Part model, mm, in its own coordinate system. Round coordinates to 2 decimals unless told otherwise and drop trailing zeros. Loops run counter-clockwise (first coordinate to the right, second up) from the corner with the lowest first, then second, coordinate; pieces in that order, holes last.
from build123d import *

# Parameters (mm, degrees)
F1_R     = 19.05
F2_DEPTH = 25.4


with BuildPart() as f2:
    # F1 (on Front) → F2 (new body)
    with BuildSketch(Plane.XZ):
        with BuildLine():
            ThreePointArc((0, 19.05), (5.579616, 5.579616), (19.05, 0))
            Line((19.05, 0), (235.130832, 0))
            ThreePointArc((235.130832, 0), (248.536825, 5.515531), (254.179965, 18.86831))
            Line((254.179965, 18.86831), (254.385811, 40.449988))
            ThreePointArc((254.385811, 40.449988), (252.162315, 49.564786), (245.857692, 56.512822))
            Line((245.857692, 56.512822), (182.583289, 98.431144))
            ThreePointArc((182.583289, 98.431144), (177.556212, 100.790591), (172.062274, 101.6))
            Line((172.062274, 101.6), (127, 101.6))
            Line((127, 101.6), (81.967876, 101.6))
            ThreePointArc((81.967876, 101.6), (76.447488, 100.782603), (71.400837, 98.400558))
            Line((71.400837, 98.400558), (8.482961, 56.455308))
            ThreePointArc((8.482961, 56.455308), (2.254099, 49.593643), (0, 40.604749))
            Line((0, 40.604749), (0, 19.05))
        make_face()
        with Locations((38.1, 29.827375)):
            Circle(F1_R, mode=Mode.SUBTRACT)
        with BuildLine():
            ThreePointArc((88.317876, 44.45), (77.477748, 39.959872), (81.967876, 50.8))
            ThreePointArc((81.967876, 50.8), (86.458004, 48.940128), (88.317876, 44.45))
        make_face(mode=Mode.SUBTRACT)
        with BuildLine():
            ThreePointArc((178.382124, 44.45), (167.541996, 39.959872), (172.032124, 50.8))
            ThreePointArc((172.032124, 50.8), (176.522252, 48.940128), (178.382124, 44.45))
        make_face(mode=Mode.SUBTRACT)
        with Locations((216.277108, 29.826619)):
            Circle(F1_R, mode=Mode.SUBTRACT)
        with BuildLine():
            ThreePointArc((138.767743, 65.500937), (116.76372, 56.856565), (127, 78.166675))
            ThreePointArc((127, 78.166675), (135.371765, 74.145309), (138.767743, 65.500937))
        make_face(mode=Mode.SUBTRACT)
        with BuildLine():
            ThreePointArc((88.317876, 82.55), (86.458004, 78.059872), (81.967876, 76.2))
            ThreePointArc((81.967876, 76.2), (77.477748, 87.040128), (88.317876, 82.55))
        make_face(mode=Mode.SUBTRACT)
        with BuildLine():
            ThreePointArc((178.412274, 82.55), (176.54173, 78.049225), (172.032124, 76.200072))
            ThreePointArc((172.032124, 76.200072), (167.582818, 87.050775), (178.412274, 82.55))
        make_face(mode=Mode.SUBTRACT)
    extrude(amount=F2_DEPTH)


solid = f2.part
1) Slice it at C-C, the plane x = 176. Give the cut face in (y, z).
Values:
outline: (-25.4, 0) - (0, 0) - (0, 39.49) - (-25.4, 39.49) - close; (-25.4, 49.41) - (0, 49.41) - (0, 77.57) - (-25.4, 77.57) - close; (-25.4, 87.53) - (0, 87.53) - (0, 101.19) - (-25.4, 101.19) - close
2) Slice it at B-B, the plane y = -7. Give the cut face in (x, z).
Values:
outline: (0, 19.05) arc R19.05 ccw to (19.05, 0) - (235.13, 0) arc R19.05 ccw to (254.18, 18.87) - (254.39, 40.45) arc R19.05 ccw to (245.86, 56.51) - (182.58, 98.43) arc R19.05 ccw to (172.06, 101.6) - (81.97, 101.6) arc R19.05 ccw to (71.4, 98.4) - (8.48, 56.46) arc R19.05 ccw to (0, 40.6) - close; hole circle Ø38.1 at (38.1, 29.83); hole circle Ø12.7 at (81.97, 44.45); hole circle Ø12.7 at (81.97, 82.55); hole (127, 78.17) arc R12.7 ccw (long way) to (138.77, 65.5) arc R12.7 ccw to start; hole circle Ø12.7 at (172.03, 44.45); hole circle Ø12.7 at (172.06, 82.55); hole circle Ø38.1 at (216.28, 29.83)
3) Wall check: line 1 along X through (y, z) = (-1.25, 25); line 2 along X through (y, z) = (-4, 82.5); line 3 along X through (y, z) = (-19.5, 44.45). Give the ranges that are in metal, low to high.
Values:
line 1: x = 0 to 19.67, 56.53 to 197.85, 234.71 to 254.24
line 2: x = 47.55 to 75.62, 88.32 to 165.71, 178.41 to 206.63
line 3: x = 0.39 to 25.89, 50.31 to 75.62, 88.32 to 165.68, 178.38 to 204.07, 228.49 to 254
4) Drop flat-ended pins along their axis: pin 1 Ø1.5 at (x, y) = (70, -19) entering from +Z; pin 2 Ø6 at (x, y) = (205.5, -11.5) entering from +Z; pin 3 Ø1 at (x, y) = (30.5, -11.5) entering from +Z. Give the stop position or say it passes through.
Values:
pin 1: stops at z = 97.97
pin 2: stops at z = 85.24
pin 3: stops at z = 71.47
5) Slice it at D-D, the plane x = 122. Give the cut face in (y, z), then the cut area to 3 significant figures.
Values:
outline: (-25.4, 0) - (0, 0) - (0, 53.47) - (-25.4, 53.47) - close; (-25.4, 77.53) - (0, 77.53) - (0, 101.6) - (-25.4, 101.6) - close
area: 1,970 mm2
6) Mould opens along X. For faces 1 (the face through (126, -13, 0)), 2 (the face through (33.97, -12.52, 11.23)), 3 (the face through (76.5, -12.5, 100.8)), 4 (the face through (234.447, -12.522, 35.549)) say: released by +X, released by -X, zero draft, split by the parting line, or undercut.
Values:
face 1: zero draft
face 2: undercut
face 3: released by -X
face 4: undercut
7) Slice it at A-A, the plane x = 38.1. Give the cut face in (y, z).
Values:
outline: (-25.4, 0) - (0, 0) - (0, 10.78) - (-25.4, 10.78) - close; (-25.4, 48.88) - (0, 48.88) - (0, 76.2) - (-25.4, 76.2) - close
